Geometry: final body of the model. Coordinates: model frame, mm. A direction names the side the tool comes from. Give positions to 0.01 mm unless a question says otherwise; leave off trailing zeros. Loops run counter-clockwise (first coordinate to the right, second up) from the corner with the lowest first, then second, coordinate; pieces in that order, holes last.
1. Section D-D, the plane z = -40. Output: boundary loops of the cut face in (x, y).
2. Access query for faces 1 (the face through (33, -6, 1)), 2 (the face through (11, -3, 28.457)), 3 (the face through (9, -3, -22.137)). Directions: +Z, -Z, +X, -X, +Y, -Y. A direction counts if a zero-diameter tool reaches every point of the face in a straight line with its end or side. Return the directions, or none.
3. Section B-B, the plane x = 52.5. Output: boundary loops of the cut face in (y, z).
4. First-contact query: P1, Ø1.8, axis at x = 16, y = -3, coming from the +Z side; P2, Ø2, axis at y = -4, z = -19.5, coming from the -X side; P3, Ø2, axis at x = 87, y = -2, coming from the +Z side. Flat tips, straight axial feed; report the tip coordinate or a pass-through.
5. Section C-C, the plane x = 81. Output: boundary loops of the cut face in (y, z).
6. Section A-A, the plane y = -3.55. Output: boundary loops of the cut face in (x, z).
7. Draft query along X for faces 4 (the face through (36.538, -2.958, 1.649)), 5 (the face through (-14.14, -2.96, 14.43)), 6 (the face through (133.725, -2.958, -5.752)), 7 (the face through (-2.38, -2.96, -10.74)). Return one class per face: +X half, -X half, draft (parallel to the pull), parting line (faces both ways), or undercut.
8. Material intervals for line 1 along Z through (x, y) = (0, -3.9); line 2 along X through (y, z) = (-0.6, -2); line 3 along X through (y, z) = (-4.75, 9.5), sorted ascending.
from build123d import *

# Parameters (mm, degrees)
F0_R     = 37.5
F0_R_2   = 11
F1_DEPTH = 6


# Not quite as in the source:
# - a feature names something its author has since deleted; it is built from what else it names


with BuildPart() as f1:
    # F0 (on Front) → F1 (new body)
    with BuildSketch(Plane.XZ):
        with BuildLine():
            ThreePointArc((18.2343609636, -22.1367832273), (85.2703314711, -58.932259595), (134.0014016628, 0))
            ThreePointArc((134.0014016628, 0), (88.6756766088, 58.1778794286), (21.1792131691, 28.4572732836))
            ThreePointArc((21.1792131691, 28.4572732836), (14.1027805373, 3.4864290135), (18.2343609636, -22.1367832273))
        make_face()
        with Locations((74.0014016628, 0)):
            Circle(F0_R, mode=Mode.SUBTRACT)
        with BuildLine():
            ThreePointArc((18.2343609636, -22.1367832273), (14.1027805373, 3.4864290135), (21.1792131691, 28.4572732836))
            Line((21.1792131691, 28.4572732836), (0, 28.4572732836))
            Line((0, 28.4572732836), (-28.6835413426, 0))
            Line((-28.6835413426, 0), (0, -22.1367832273))
            Line((0, -22.1367832273), (18.2343609636, -22.1367832273))
        make_face()
        Circle(F0_R_2, mode=Mode.SUBTRACT)
    extrude(amount=F1_DEPTH)


solid = f1.part
Answers below:
1. outline: (29.28, -6) - (118.72, -6) - (118.72, 0) - (29.28, 0) - close
2. face 1: +Z, -Z, +X, -X, -Y
2. face 2: +Z, -X, +Y, -Y
2. face 3: -Z, -X, +Y, -Y
3. outline: (-6, -56.02) - (0, -56.02) - (0, -30.72) - (-6, -30.72) - close; (-6, 30.72) - (0, 30.72) - (0, 56.02) - (-6, 56.02) - close
4. P1: stops at z = 28.46
4. P2: stops at x = -4.71
4. P3: stops at z = 58.79
5. outline: (-6, -59.59) - (0, -59.59) - (0, -36.84) - (-6, -36.84) - close; (-6, 36.84) - (0, 36.84) - (0, 59.59) - (-6, 59.59) - close
6. outline: (-28.68, 0) - (0, -22.14) - (18.23, -22.14) arc R60 ccw (long way) to (21.18, 28.46) - (0, 28.46) - close; hole circle Ø22 at (0, 0); hole circle Ø75 at (74, 0)
7. face 4: undercut
7. face 5: -X half
7. face 6: parting line
7. face 7: undercut
8. line 1: z = -22.14 to -11, 11 to 28.46
8. line 2: x = -26.09 to -10.82, 10.82 to 36.55, 111.45 to 133.97
8. line 3: x = -19.11 to -5.55, 5.55 to 37.72, 110.28 to 133.24
